Geometry: see drawing. Coordinates: mm, zero at the bounding-box minimum. A direction names the side the tool comes from. Coordinates: 2 decimals unless noted, no trailing zeros. Loops run counter-clockwise (first coordinate to the right, second up) from the corner with the lowest first, then second, coordinate; pieces in that order, holes last. Notation, with made-up numbers: (22, -36) -> (29, -36) arc R24 ccw to (29, -10) -> close; hole circle Ø6 at (49, -23). An arc over 180 degrees is marked (long way). One line per item, written item: value. Start each with the question number.
Item 1: Contact query for flat-ended pins moving along their axis: pin 1 Ø3 at (y, z) = (11, 44.5) entering from +X; pin 2 Ø2 at (x, y) = (19, 8.5) entering from -Z; pin 3 Ø15 at (x, z) = (50.5, 41.5) entering from -Y. Output: stop coordinate, or through.
Item 2: Section query C-C on y = 4.5. Return loops of the section in (x, z), then the cut area to 3 significant figures.
Item 3: Ray query, probe 1 along X at (y, z) = (10.25, 38.1) (3 decimals); probe 2 along Y at (x, z) = (23, 35); probe 3 along Z at (x, y) = (60, 1.75). Return the intervals inside material, ascending. Write a range as from..to.
Item 4: Section query A-A on z = 38.1. Return loops of the section in (x, y) (3 decimals).
Item 5: Set-up query: the marked faces 1 and 2. Return all of +Z, -Z, +X, -X, +Y, -Y with unobstructed straight access to the full face (end or side cutting, diameter ignored); none if empty.
Item 6: Mould query, pull axis Z, two halves, no side actions, for the marked faces 3, 4 and 5. Classes: +Z half, -Z half, draft (parallel to the pull), parting line (faces both ways), or undercut.
Item 7: Section query B-B on x = 38.1. Return loops of the section in (y, z) (3 decimals).
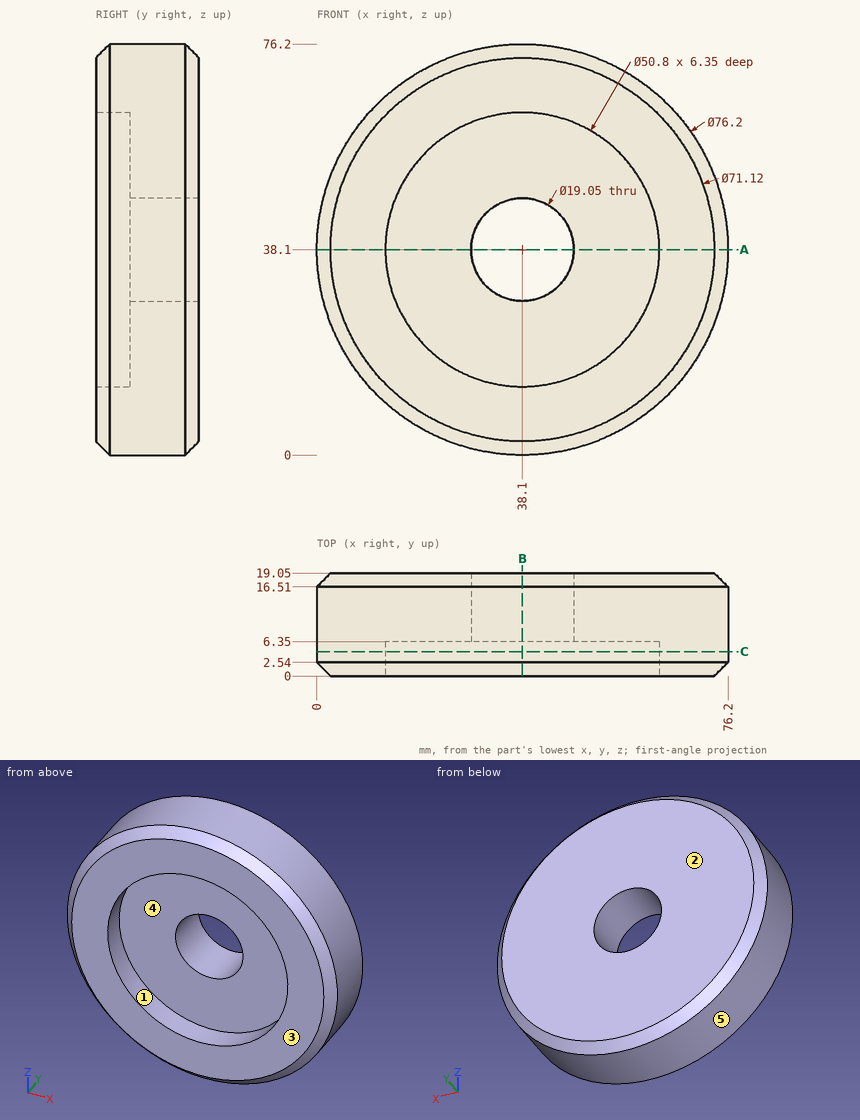
Reply:
1. pin 1: stops at x = 75.88
1. pin 2: stops at z = 4.57
1. pin 3: stops at y = 6.35
2. outline: circle Ø76.2 at (38.1, 38.1); hole circle Ø50.8 at (38.1, 38.1)
2. area: 2,530 mm²
3. probe 1: x = 0..28.575, 47.625..76.2
3. probe 2: y = 6.35..19.05
3. probe 3: z = 7.89..25.23, 50.97..68.31
4. outline: (0, 2.54) -> (2.54, 0) -> (12.7, 0) -> (12.7, 6.35) -> (28.575, 6.35) -> (28.575, 19.05) -> (2.54, 19.05) -> (0, 16.51) -> close; (47.625, 6.35) -> (63.5, 6.35) -> (63.5, 0) -> (73.66, 0) -> (76.2, 2.54) -> (76.2, 16.51) -> (73.66, 19.05) -> (47.625, 19.05) -> close
5. face 1: -Y
5. face 2: +Z, -Z, +X, -X, +Y
6. face 3: draft
6. face 4: undercut
6. face 5: parting line
7. outline: (0, 2.54) -> (2.54, 0) -> (16.51, 0) -> (19.05, 2.54) -> (19.05, 28.575) -> (6.35, 28.575) -> (6.35, 12.7) -> (0, 12.7) -> close; (0, 63.5) -> (6.35, 63.5) -> (6.35, 47.625) -> (19.05, 47.625) -> (19.05, 73.66) -> (16.51, 76.2) -> (2.54, 76.2) -> (0, 73.66) -> close
